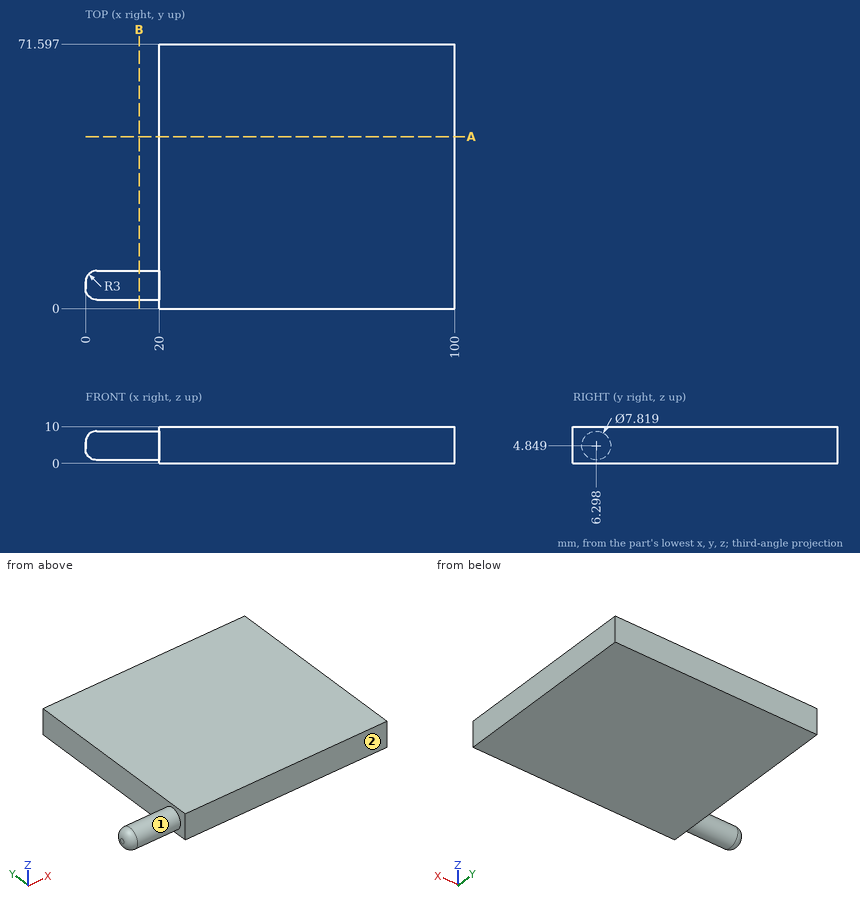
Design review of the part shown in the three views and the two pictorial views. Dimensions are in mm from the part's minimum x, y and z. A direction names the side the tool comes from. Coordinates: 2 decimals unless noted, no trailing zeros. Order: outer loops, then holes, each group sorted by start corner. A loop starts at its lowest first (then second) coordinate and runs counter-clockwise, first axis right, second up.
1) For the marked faces 1 and 2, list the 3-axis set-ups (+Z, -Z, +X, -X, +Y, -Y) from which the entire face can be reached by the end or side of a thin tool; tool diameter is ignored.
2) Take a section at A-A, the plane y = 46.5. Give the boundary of the cut face in (x, z), and give its area (3 significant figures).
3) Take a section at B-B, the plane x = 14.5. Give the boundary of the cut face in (y, z), and give its area (3 significant figures).
4) Clearance check with flat-ended pins moving along their axes: pin 1 (3 mm diameter, centred on y = 22, z = 7.5, fed in from -X); pin 2 (5 mm diameter, centred on x = 10.5, z = 5.5, fed in from -Y). State where each tip first meets the part, or that it passes through.
5) Wall thickness on line 1 along X through (y, z) = (16.5, 7.5); line 2 along Y through (x, z) = (4, 8.25) (1 decimal); line 3 along Y through (x, z) = (11.5, 4) (1 decimal): over which ranges is each line inside the solid? List them lowest first.
Returned:
1. face 1: -X
1. face 2: +Z, -Z, +X, -X, -Y
2. outline: (20, 0) - (100, 0) - (100, 10) - (20, 10) - close
2. area: 800 mm2
3. outline: circle Ø7.82 at (6.3, 4.85)
3. area: 48.0 mm2
4. pin 1: stops at x = 20
4. pin 2: stops at y = 2.39
5. line 1: x = 20 to 100
5. line 2: y = 4.4 to 8.2
5. line 3: y = 2.5 to 10.1
